from build123d import *

# Parameters (mm, degrees)
F1_DEPTH       = 9.525
F2_D           = 5.6134
F2_DEPTH       = 9.525
F2_CBORE_D     = 8.255
F2_CBORE_DEPTH = 4.826


with BuildPart() as f1:
    # F0 (on Front) → F1 (new body)
    with BuildSketch(Plane.XZ):
        Polygon((30.1625, 19.05), (-68.2625, 19.05), (-68.2625, -19.05), (68.2625, -19.05), (68.2625, 19.05), align=None)
    extrude(amount=F1_DEPTH)

    # F2
    with Locations(Plane(origin=(0, 0, 0), x_dir=(1, 0, 0), z_dir=(0, 1, 0))):
        with Locations((-63.1825, 14.2875), (-63.1825, -14.2875), (63.1825, -14.2875), (63.1825, 14.2875)):
            CounterBoreHole(F2_D / 2, F2_CBORE_D / 2, F2_CBORE_DEPTH, depth=F2_DEPTH)


solid = f1.part
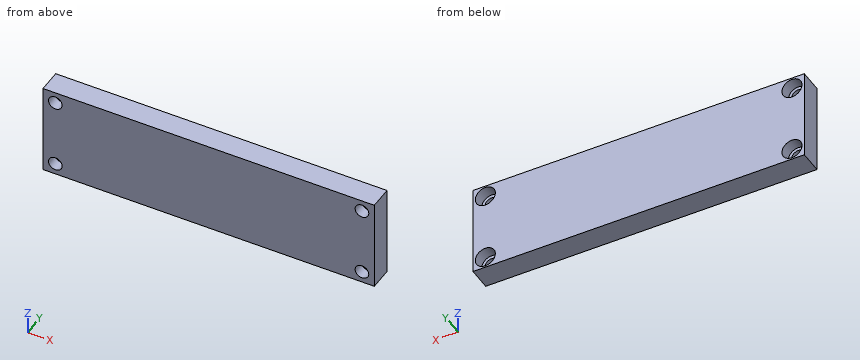
Input: part model. Units: mm. Frame: model coordinates. Give positions to 0.01 mm unless a question says otherwise; leave off trailing zeros. Order: outer loops, then holes, each group sorted by start corner. A loop starts at its lowest first (then second) coordinate and runs counter-clockwise, first axis right, second up. Notation, with made-up numbers: M -26,-22 L -11,-22 A6 cw -11,-14 Z; hole C 13,-33 d10. An arc over 180 degrees is marked long. Answer as a JSON object with one key per item and string values.
1. First-contact query: P1, Ø7.5, axis at x = -63.18, z = 14.29, coming from the +Y side; P2, Ø2.5, axis at x = 64, z = 15.5, coming from the +Y side. Flat tips, straight axial feed; report the tip coordinate or a pass-through.
Result sheet:
{"P1": "y = -4.83", "P2": "through"}
2. Ray query, line 1 (Z direction, x = -60.5, y = -2.25); line 2 (X direction, y = -4.75, z = -14.5); line 3 (X direction, y = -2.75, z = -13.5). Return the intervals inside material, ascending. Write a range as [from, to].
Result sheet:
{"line 1": "[-19.05, -17.42], [-11.15, 11.15], [17.42, 19.05]", "line 2": "[-68.26, -67.3], [-59.06, 59.06], [67.3, 68.26]", "line 3": "[-68.26, -67.23], [-59.13, 59.13], [67.23, 68.26]"}
3. Cut plane B-B, the plane y = -2. State how many separate pieces and enclosed holes the cut face has, and give its area (3 significant figures).
Result sheet:
{"separate pieces": "1", "enclosed holes": "4", "area": "4,990 mm²"}
4. Cut plane A-A, the plane y = -7.5. Output: boundary loops of the cut face in (x, z), and give its area (3 significant figures).
Result sheet:
{"outline": "M -68.26,-19.05 L 68.26,-19.05 L 68.26,19.05 L -68.26,19.05 Z; hole C -63.18,-14.29 d5.61; hole C -63.18,14.29 d5.61; hole C 63.18,-14.29 d5.61; hole C 63.18,14.29 d5.61", "area": "5,100 mm²"}
